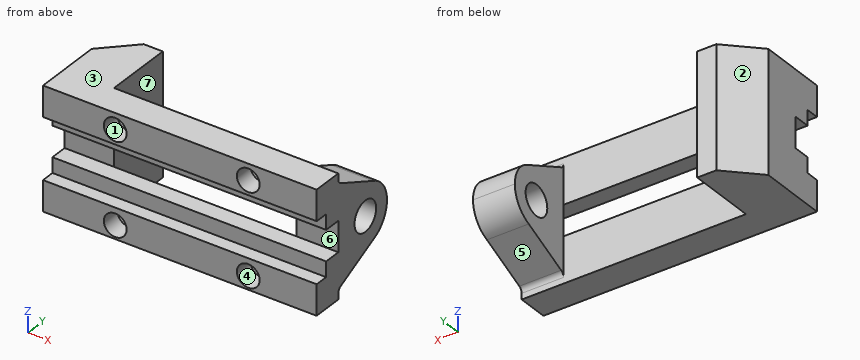
from build123d import *

# Parameters (mm, degrees)
SKETCH1_W                  = 144
SKETCH1_H                  = 64
BOSS_EXTRUDE1_DEPTH        = 16
SKETCH2_W                  = 26
SKETCH2_H                  = 64
BOSS_EXTRUDE2_DEPTH        = 36
CUT_EXTRUDE1_DEPTH         = 1
CUT_EXTRUDE1_DEPTH_BACK    = 65
SKETCH4_W                  = 22
SKETCH4_H                  = 64
BOSS_EXTRUDE3_DEPTH        = 36
CUT_EXTRUDE2_DEPTH         = 1
CUT_EXTRUDE2_DEPTH_BACK    = 145
SKETCH6_R                  = 8
CUT_EXTRUDE3_DEPTH         = 36
F_12_0MM_DOWEL_HOLE1_D     = 12
F_12_0MM_DOWEL_HOLE1_DEPTH = 10
F_12_0MM_DOWEL_HOLE1_TIP   = 3.605163714


with BuildPart() as part:
    # Sketch1 → Boss-Extrude1 (new body)
    with BuildSketch(Plane(origin=(0, 0, 0), x_dir=(1, 0, 0), z_dir=(0, 1, 0))):
        Rectangle(SKETCH1_W, SKETCH1_H)
    extrude(amount=BOSS_EXTRUDE1_DEPTH)

    # Sketch2 → Boss-Extrude2 (add)
    with BuildSketch(Plane(origin=(0, 16, 0), x_dir=(1, 0, 0), z_dir=(0, 1, 0))):
        with Locations((-59, 0)):
            Rectangle(SKETCH2_W, SKETCH2_H)
    extrude(amount=BOSS_EXTRUDE2_DEPTH)

    # Sketch3 → Cut-Extrude1 (cut, two sides)
    with BuildSketch(Plane.XY.offset(32)) as cut_extrude1_sk:
        Polygon((-72, 36), (-56, 52), (-72, 52), align=None)
    extrude(amount=CUT_EXTRUDE1_DEPTH, mode=Mode.SUBTRACT)
    extrude(cut_extrude1_sk.sketch, amount=-CUT_EXTRUDE1_DEPTH_BACK, mode=Mode.SUBTRACT)

    # Sketch4 → Boss-Extrude3 (add)
    with BuildSketch(Plane(origin=(0, 16, 0), x_dir=(1, 0, 0), z_dir=(0, 1, 0))):
        with Locations((61, 0)):
            Rectangle(SKETCH4_W, SKETCH4_H)
    extrude(amount=BOSS_EXTRUDE3_DEPTH)

    # Sketch5 → Cut-Extrude2 (cut, two sides)
    with BuildSketch(Plane(origin=(72, 0, 0), x_dir=(0, 0, -1), z_dir=(1, 0, 0))) as cut_extrude2_sk:
        Polygon((-16, 7), (-16, 0), (16, 0), (16, 7), (8, 7), (8, 16), (-8, 16), (-8, 7), align=None)
    extrude(amount=CUT_EXTRUDE2_DEPTH, mode=Mode.SUBTRACT)
    extrude(cut_extrude2_sk.sketch, amount=-CUT_EXTRUDE2_DEPTH_BACK, mode=Mode.SUBTRACT)

    # Sketch6 → Cut-Extrude3 (cut)
    with BuildSketch(Plane(origin=(72, 0, 0), x_dir=(0, 0, -1), z_dir=(1, 0, 0))):
        with BuildLine():
            Line((-32, 52), (-32, 16))
            Line((-32, 16), (-28.843717868, 16))
            ThreePointArc((-28.843717868, 16), (-27.231819043, 16.469825663), (-26.124794507, 17.732145215))
            Line((-26.124794507, 17.732145215), (-14.958449756, 41.678448811))
            ThreePointArc((-14.958449756, 41.678448811), (-9.086936164, 49.169190983), (8.8e-08, 52))
            Line((8.8e-08, 52), (-32, 52))
        make_face()
        with Locations((0, 36)):
            Circle(SKETCH6_R)
        with BuildLine():
            Line((32, 52), (8.8e-08, 52))
            ThreePointArc((8.8e-08, 52), (9.086936237, 49.169190933), (14.958449756, 41.678448811))
            Line((14.958449756, 41.678448811), (26.124794507, 17.732145215))
            ThreePointArc((26.124794507, 17.732145215), (27.231819043, 16.469825663), (28.843717868, 16))
            Line((28.843717868, 16), (32, 16))
            Line((32, 16), (32, 52))
        make_face()
    extrude(amount=-CUT_EXTRUDE3_DEPTH, mode=Mode.SUBTRACT)

    # Ø12.0mm Dowel Hole1
    with Locations(Plane(origin=(0, 0, 0), x_dir=(-1, 0, 0), z_dir=(0, -1, 0))):
        with Locations((34, -23.551834062), (-36, -23.551834062), (-36, 24.957913708), (34, 24.957913708)):
            Hole(F_12_0MM_DOWEL_HOLE1_D / 2, depth=F_12_0MM_DOWEL_HOLE1_DEPTH)
            with Locations((0, 0, -(F_12_0MM_DOWEL_HOLE1_DEPTH + F_12_0MM_DOWEL_HOLE1_TIP / 2))):  # 118° drill point
                Cone(0, F_12_0MM_DOWEL_HOLE1_D / 2, F_12_0MM_DOWEL_HOLE1_TIP, mode=Mode.SUBTRACT)


solid = part.part
Geometry check sheet. Reference: the model listing, model coordinates, mm. Face numbers are marked on the shaded views. A direction names the side the tool comes from. Round coordinates to 2 decimals unless told otherwise and drop trailing zeros. Order: outer loops, then holes, each group sorted by start corner. A loop starts at its lowest first (then second) coordinate and runs counter-clockwise, first axis right, second up. Notation, with made-up numbers: (76, 61) -> (80, 61) arc R24 ccw to (80, 77) -> close; hole circle Ø2 at (34.25, 46). An arc over 180 degrees is marked (long way). Use one line per item in the form item = value.
1. Mould release check, pull along X, two halves, no side actions. Record for the marked faces 1, 2 and 3: pulls with the +X half, pulls with the -X half, needs draft (parallel to the pull), parting line crosses it, or undercut.
Working result:
face_1 = undercut
face_2 = pulls with the -X half
face_3 = needs draft
2. Scan lines: line 1 along Z through (x, y) = (-34, 4); line 2 along Z through (x, y) = (-34, 8); line 3 along Z through (x, y) = (-5.5, 9). Record each from-to range of solid material in increasing order. Write a range as from..to.
Working result:
line_1 = -32..-30.96, -18.96..-16, 16..17.55, 29.55..32
line_2 = -32..-30.96, -18.96..-8, 8..17.55, 29.55..32
line_3 = -32..-8, 8..32
3. Cross-section at A-A, the plane x = -26. Enter the section's corners in (y, z), plus the area to 3 significant figures.
Working result:
outline = (0, -32) -> (16, -32) -> (16, -8) -> (7, -8) -> (7, -16) -> (0, -16) -> close; (0, 16) -> (7, 16) -> (7, 8) -> (16, 8) -> (16, 32) -> (0, 32) -> close
area = 656 mm^2
4. Cross-section at C-C, the plane z = -5. Enter the section's corners in (x, y) (3 decimals), plus the area to 3 significant figures.
Working result:
outline = (-72, 16) -> (-46, 16) -> (-46, 52) -> (-56, 52) -> (-72, 36) -> close; (50, 16) -> (72, 16) -> (72, 29.755) -> (50, 29.755) -> close; (50, 42.245) -> (72, 42.245) -> (72, 51.199) -> (50, 51.199) -> close
area = 1,310 mm^2
5. Go/stop test with flat-tipped pins: pin 1 (14 mm diameter, centred on x = -34, z = 23.55, fed in from +Y); pin 2 (4 mm diameter, centred on x = -18, z = 10.5, fed in from -Y); pin 3 (5 mm diameter, centred on x = 56.5, z = -3, fed in from -Y). Record where each tip stops, or that it passes through.
Working result:
pin_1 = 16
pin_2 = 7
pin_3 = 16
6. Set-up check for the marked faces 4, 5, 6 and 7: record each of +Z, -Z, +X, -X, +Y, -Y from which the full face is reachable in a straight line by a thin tool's end or side.
Working result:
face_4 = -Y
face_5 = -Z, +X, +Y
face_6 = +X, -X, -Y
face_7 = +Z, -Z, +Y
7. Cross-section at B-B, the plane y = 46. Enter the section's corners in (x, z).
Working result:
outline = (-62, -32) -> (-46, -32) -> (-46, 32) -> (-62, 32) -> close; (50, -12.49) -> (72, -12.49) -> (72, 12.49) -> (50, 12.49) -> close
8. Cross-section at D-D, the plane y = 39. Enter the section's corners in (x, z), plus the area to 3 significant figures.
Working result:
outline = (-69, -32) -> (-46, -32) -> (-46, 32) -> (-69, 32) -> close; (50, -16.21) -> (72, -16.21) -> (72, -7.42) -> (50, -7.42) -> close; (50, 7.42) -> (72, 7.42) -> (72, 16.21) -> (50, 16.21) -> close
area = 1,860 mm^2
